```python
from build123d import *

# Parameters (mm, degrees)
SKETCH062_R  = 1.25
PAD029_DEPTH = 1.8
SKETCH064_R  = 1.25
PAD032_DEPTH = 3
FILLET004_R  = 2


with BuildPart() as part:
    # Sketch062 → Pad029 (new body, symmetric)
    with BuildSketch(Plane.YZ.offset(-41.1)):
        with BuildLine():
            Line((96.000005, 10.999996), (100.999998, 10.999996))
            Line((100.999998, 10.999996), (100.999998, 27))
            Line((100.999998, 27), (92.999998, 17.465971))
            Line((92.999998, 14), (92.999998, 17.465971))
            ThreePointArc((92.999998, 14), (93.878624, 11.87862), (96.000005, 10.999996))
        make_face()
        with Locations((97, 15)):
            Circle(SKETCH062_R, mode=Mode.SUBTRACT)
    extrude(amount=PAD029_DEPTH, both=True)

    # Sketch064 (on Face7 of Clone022) → Pad032 (new body)
    with BuildSketch(Plane(origin=(-42.9, 0, 0), x_dir=(0, -1, 0), z_dir=(-1, 0, 0))):
        with BuildLine():
            Line((-100.999998, 27), (-92.999998, 17.465971))
            Line((-92.999998, 17.465971), (-92.999998, 14))
            ThreePointArc((-96.000005, 10.999996), (-93.87868, 11.878676), (-92.999998, 14))
            Line((-96.000005, 10.999996), (-100.999998, 10.999996))
            Line((-100.999998, 10.999996), (-100.999998, 27))
        make_face()
        with Locations((-97, 15)):
            Circle(SKETCH064_R, mode=Mode.SUBTRACT)
    extrude(amount=PAD032_DEPTH)

    # Fillet004
    fillet004_edges = [part.edges().sort_by_distance(p)[0] for p in [
        (-45.9, 98.500001, 10.999996),
        (-45.9, 93.87868, 11.878676),
        (-45.9, 92.999998, 15.732986),
        (-45.9, 96.999998, 22.232986),
    ]]
    fillet(fillet004_edges, radius=FILLET004_R)


with BuildPart() as part_1:
    # Body045 placement: moved
    add(part.part.moved(Location((82.2, 0, 0))))


solid = part_1.part
```
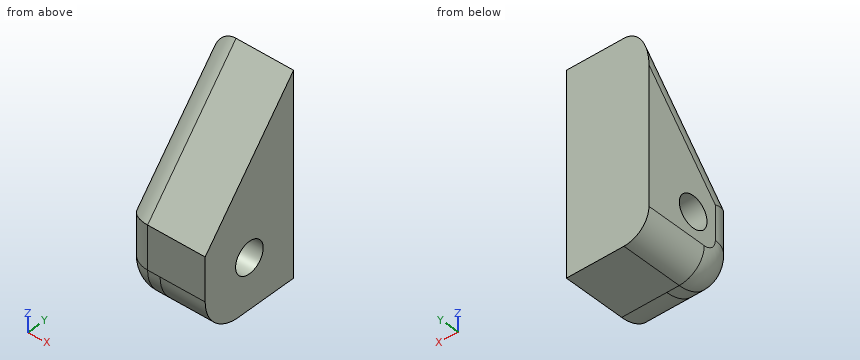
CAD build for the part. Positions are in the model's coordinates, mm. Coordinates: 2 decimals unless noted, no trailing zeros. Order: outer loops, then holes, each group sorted by start corner. A loop starts at its lowest first (then second) coordinate and runs counter-clockwise, first axis right, second up. Notation, with made-up numbers: M 17,9.25 L 22,9.25 A13 ccw 22,31.25 Z; hole C 14.25,-9.5 d9. An arc over 180 degrees is marked long. Answer as CSV lines item,"result".
1) Drill centre lines: L1, parallel to Y at x = 42.1, z = 15; L2, parallel to Z at x = 41.8, y = 97; L3, parallel to Z at x = 37.55, y = 97. Where is each one in solid material? Low to high. Write a range as from..to.
Verdict:
L1,"93..95.75, 98.25..101"
L2,"11..13.75, 16.25..22.23"
L3,"11.15..13.75, 16.25..22.01"
2) Cut at A-A (z = 15). List the corners of the cut face in (x, y), then the cut area to 3 significant figures.
Verdict:
outline,"M 36.3,95 A2 ccw 38.3,93 L 42.9,93 L 42.9,95.75 L 36.3,95.75 Z; M 36.3,98.25 L 42.9,98.25 L 42.9,101 L 36.3,101 Z"
area,"35.4 mm2"
3) Flat gauge pins, fed straight in: P1, Ø2, axis at y = 97, z = 15, coming from the -X side; P2, Ø2, axis at x = 42, y = 99, coming from the +Z side; P3, Ø1.5, axis at x = 38.5, z = 24, coming from the -Y side; P4, Ø1.5, axis at y = 95, z = 12, coming from the -X side. Where does each tip first touch, or does it go through?
Verdict:
P1,"through"
P2,"z = 25.81"
P3,"y = 97.85"
P4,"x = 36.36"
4) Cut at B-B (x = 42.5). List the corners of the cut face in (y, z), then the cut area to 3 significant figures.
Verdict:
outline,"M 93,14 A3 ccw 96,11 L 101,11 L 101,27 L 93,17.47 Z; hole C 97,15 d2.5"
area,"83.0 mm2"
